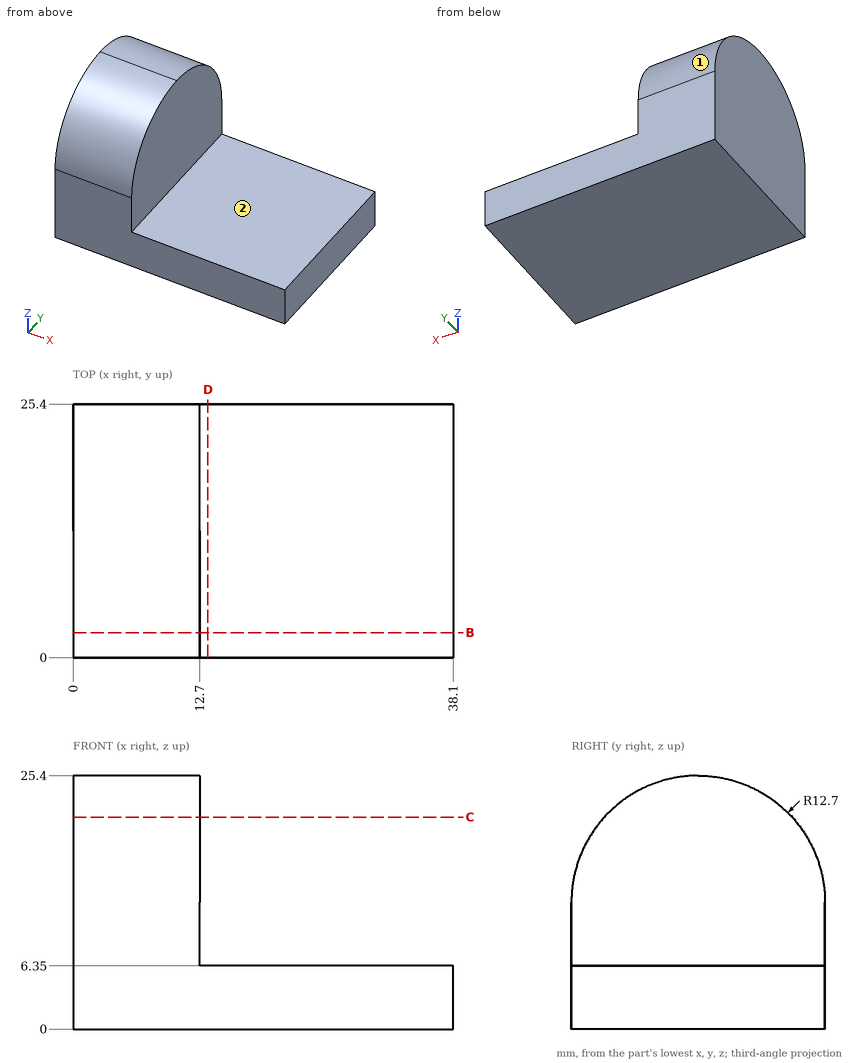
Input: dimensioned drawing with shaded views. Units: mm. Origin: part minimum x, y, z. A direction names the side the tool comes from. Round coordinates to 2 decimals unless told otherwise and drop trailing zeros. Order: outer loops, then holes, each group sorted by start corner. A loop starts at its lowest first (then second) coordinate and runs counter-clockwise, first axis right, second up.
1. Cut plane B-B, the plane y = 2.5. Output: boundary loops of the cut face in (x, z), then the cut area to 3 significant figures.
The answers:
outline: (0, 0) - (38.1, 0) - (38.1, 6.35) - (12.7, 6.35) - (12.7, 20.27) - (0, 20.27) - close
area: 419 mm2
2. Cut plane C-C, the plane z = 21.25. Output: boundary loops of the cut face in (x, y).
The answers:
outline: (0, 3.31) - (12.7, 3.31) - (12.7, 22.09) - (0, 22.09) - close
3. Cut plane D-D, the plane x = 13.5. Output: boundary loops of the cut face in (y, z), then the cut area to 3 significant figures.
The answers:
outline: (0, 0) - (25.4, 0) - (25.4, 6.35) - (0, 6.35) - close
area: 161 mm2
4. Pin query (flat end, axial travel): P1, Ø5, axis at x = 13.5, y = 20.5, coming from the +Z side; P2, Ø3, axis at x = 13.5, y = 21, coming from the +Z side; P3, Ø8, axis at x = 24, y = 3.5, coming from the +Z side. Return the tip coordinate at first contact, or that it passes through.
The answers:
P1: stops at z = 24.18
P2: stops at z = 23.28
P3: stops at z = 6.35
5. Material intervals for line 1 (Z direction, x = 19, y = 22.5); line 2 (X direction, y = 4, z = 16.75); line 3 (Z direction, x = 12, y = 19.25), sorted ascending.
The answers:
line 1: z = 0 to 6.35
line 2: x = 0 to 12.7
line 3: z = 0 to 23.58
6. Set-up query: the marked faces 1 and 2. Return all of +Z, -Z, +X, -X, +Y, -Y with unobstructed straight access to the full face (end or side cutting, diameter ignored); none if empty.
The answers:
face 1: +Z, +X, -X, +Y
face 2: +Z, +X, +Y, -Y
